Part print with two shaded views. Sizes in mm from the minimum x, y, z corner. A direction names the side the tool comes from. Round coordinates to 2 decimals unless told otherwise and drop trailing zeros. Write each loop counter-clockwise with the first axis right and the second up, starting at its lowest first coordinate (ties: lowest second). Pieces come first, ordered by that corner, then holes. Notation, with made-up numbers: (82.5, 49.25) - (97.5, 49.25) arc R17 cw to (97.5, 59.25) - close; hole circle Ø8 at (24, 19). An arc over 180 degrees is marked (long way). Answer as a JSON object with one key per item and string values. Group by question number.
Item 1: Two-plate mould, pull along X, no slides. Class the marked faces 1, 2, 3 and 4: +X half, -X half, draft (parallel to the pull), parting line (faces both ways), or undercut.
Item 2: Slice it at A-A, the plane x = 1.75. List the corners of the cut face in (y, z).
Item 3: Probe line 1 (Z direction, x = 1.75, y = 16.25); line 2 (Y direction, x = 11, z = 11); line 3 (X direction, y = 6, z = 2.25). List the from-to ranges inside material, lowest first. Write a range as from..to.
Item 4: Slice it at D-D, the plane y = 17.5. List the corners of the cut face in (x, z).
Item 5: Flat gauge pins, fed straight in: pin 1 (1 mm diameter, centred on x = 28.5, y = 20.5, fed in from +Z); pin 2 (4 mm diameter, centred on y = 20, z = 3.5, fed in from -X); pin 3 (4 mm diameter, centred on y = 24.5, z = 5.5, fed in from +X); pin 4 (5 mm diameter, centred on x = 15.5, y = 26, fed in from -Z). Where does each tip first touch, or does it go through?
Item 6: Slice it at C-C, the plane z = 4. List the corners of the cut face in (x, y).
Item 7: Which spindle directions (+Z, -Z, +X, -X, +Y, -Y) get a long thin tool onto all of the face, cutting with end or side? Do the marked faces 5, 6, 7 and 8. Say none if no direction does.
Item 8: Slice it at B-B, the plane x = 14.5. List the corners of the cut face in (y, z), then the cut area to 3 significant figures.
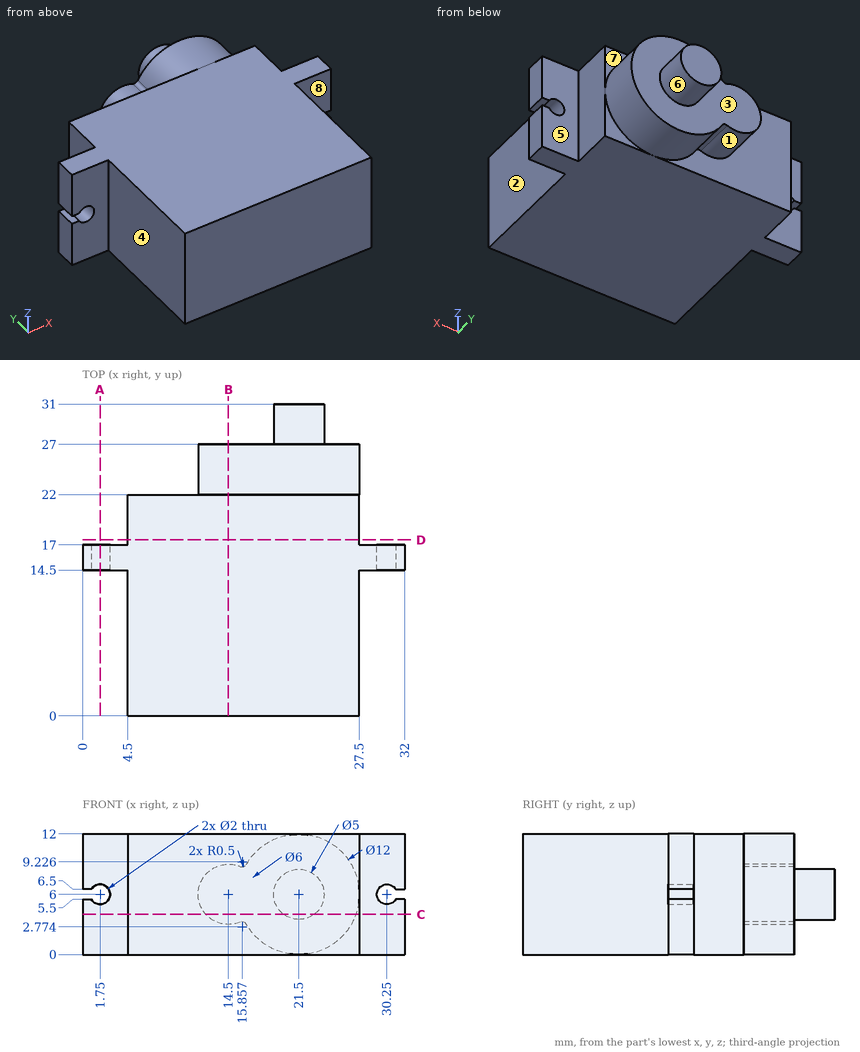
Geometry says:
{
 "1": {"face 1": "undercut", "face 2": "+X half", "face 3": "draft", "face 4": "-X half"},
 "2": {"outline": "(14.5, 0) - (17, 0) - (17, 5) - (14.5, 5) - close; (14.5, 7) - (17, 7) - (17, 12) - (14.5, 12) - close"},
 "3": {"line 1": "z = 0..5, 7..12", "line 2": "y = 0..22", "line 3": "x = 4.5..27.5"},
 "4": {"outline": "(4.5, 0) - (27.5, 0) - (27.5, 12) - (4.5, 12) - close"},
 "5": {"pin 1": "passes through", "pin 2": "stops at x = 4.5", "pin 3": "stops at x = 27.5", "pin 4": "stops at z = 1.13"},
 "6": {"outline": "(0, 14.5) - (4.5, 14.5) - (4.5, 0) - (27.5, 0) - (27.5, 14.5) - (32, 14.5) - (32, 17) - (27.5, 17) - (27.5, 22) - (27.16, 22) - (27.16, 27) - (23, 27) - (23, 31) - (20, 31) - (20, 27) - (12.26, 27) - (12.26, 22) - (4.5, 22) - (4.5, 17) - (0, 17) - close"},
 "7": {"face 5": "+Z, -Z, +X, +Y", "face 6": "+Y", "face 7": "+Z, +X, +Y", "face 8": "+Z, -Z, +X, -Y"},
 "8": {"outline": "(0, 0) - (22, 0) - (22, 3) - (27, 3) - (27, 9) - (22, 9) - (22, 12) - (0, 12) - close", "area": "294 mm^2"}
}
